from build123d import *

# Parameters (mm, degrees)
F0_R     = 3
F0_R_2   = 2.5
F0_R_3   = 2.25
F1_DEPTH = 3.1


with BuildPart() as f1:
    # F0 (on Top) → F1 (new body)
    with BuildSketch(Plane.XY):
        with BuildLine():
            ThreePointArc((29.159625, -4.46566), (32.476252, 0.673465), (34.084613, 6.574635))
            Line((34.084613, 6.574635), (34.084613, 11.068079))
            ThreePointArc((34.084613, 11.068079), (28.342014, 22.974813), (16.426098, 28.698335))
            Line((16.426098, 28.698335), (11.996317, 28.698335))
            ThreePointArc((11.996317, 28.698335), (-3.833381, 17.446484), (-2.647776, -1.938506))
            Line((-2.647776, -1.938506), (29.159625, -4.46566))
        make_face()
        with Locations((-0.443478, 2.051086)):
            Circle(F0_R, mode=Mode.SUBTRACT)
        with Locations((27.368436, -0.239537)):
            Circle(F0_R, mode=Mode.SUBTRACT)
        with Locations((-0.025214, 15.76334)):
            Circle(F0_R_2, mode=Mode.SUBTRACT)
        with Locations((14.211208, 8.821357)):
            Circle(F0_R_3, mode=Mode.SUBTRACT)
        with Locations((29.20861, 13.34557)):
            Circle(F0_R_2, mode=Mode.SUBTRACT)
        with Locations((15.398228, 25.120057)):
            Circle(F0_R, mode=Mode.SUBTRACT)
    extrude(amount=F1_DEPTH)


solid = f1.part
Part model, mm, in its own coordinate system. Give positions to 0.01 mm unless a question says otherwise; leave off trailing zeros. Loops run counter-clockwise (first coordinate to the right, second up) from the corner with the lowest first, then second, coordinate; pieces in that order, holes last.
(1) Drill centre lines: line 1 along Y through (x, z) = (14.5, 2.45); line 2 along Y through (x, z) = (27, 2.7); line 3 along X through (y, z) = (1, 0.2). Where is each one in solid material? Low to high.
Return value:
line 1: y = -3.3 to 6.59, 11.05 to 22.26, 27.98 to 28.7
line 2: y = -4.29 to -3.22, 2.74 to 12.17, 14.52 to 24.2
line 3: x = -4.2 to -3.25, 2.37 to 24.64, 30.1 to 32.62
(2) Pin check, flat tips, straight feed: pin 1 (1 mm diameter, centred on x = 3.5, z = 2.5, fed in from +Y); pin 2 (3.5 mm diameter, centred on x = 15.4, y = 25.12, fed in from +Z); pin 3 (1 mm diameter, centred on y = 20.5, z = 2.5, fed in from +X); pin 4 (1.5 mm diameter, centred on y = 16.5, z = 2.5, fed in from -X). Stop position of each tip, or through.
Return value:
pin 1: stops at y = 26.02
pin 2: passes through
pin 3: stops at x = 30.8
pin 4: stops at x = -4.55
(3) Pull direction Y, two halves, no side cores. Call faces 1 (the flat face through (14, 28.698, 2)), 2 (the cylindrical face through (1.17, 4.58, 1.53)), 3 (the cylindrical face through (13.723, 6.625, 1.528)), 4 (the cylindrical face through (32.441, 0.595, 1.528)): pulls with the +Y half, pulls with the -Y half, needs draft (parallel to the pull), parting line crosses it, or undercut.
Return value:
face 1: pulls with the +Y half
face 2: undercut
face 3: undercut
face 4: pulls with the -Y half
(4) Band-saw the part on C-C (z = 1.5). Write the cut outline in (x, y).
Return value:
outline: (-2.65, -1.94) - (29.16, -4.47) arc R20 ccw to (34.08, 6.57) - (34.08, 11.07) arc R20 ccw to (16.43, 28.7) - (12, 28.7) arc R20 ccw to start; hole circle Ø6 at (-0.44, 2.05); hole circle Ø5 at (-0.03, 15.76); hole circle Ø4.5 at (14.21, 8.82); hole circle Ø6 at (15.4, 25.12); hole circle Ø6 at (27.37, -0.24); hole circle Ø5 at (29.21, 13.35)
(5) Band-saw the part on A-A (y = 16.5). Write the cut outline in (x, z).
Return value:
outline: (-4.26, 0) - (-2.41, 0) - (-2.41, 3.1) - (-4.26, 3.1) - close; (2.36, 0) - (32.68, 0) - (32.68, 3.1) - (2.36, 3.1) - close
(6) Band-saw the part on D-D (x = 3). Write the cut outline in (y, z), and give its area (3 significant figures).
Return value:
outline: (-2.39, 0) - (25.38, 0) - (25.38, 3.1) - (-2.39, 3.1) - close
area: 86.1 mm2
(7) Band-saw the part on B-B (x = 17). Write the cut outline in (y, z), and give its area (3 significant figures).
Return value:
outline: (-3.5, 0) - (22.58, 0) - (22.58, 3.1) - (-3.5, 3.1) - close; (27.66, 0) - (28.63, 0) - (28.63, 3.1) - (27.66, 3.1) - close
area: 83.9 mm2
